Model file for the job. Use its own axes, mm. Round coordinates to 2 decimals unless told otherwise and drop trailing zeros. Loops run counter-clockwise (first coordinate to the right, second up) from the corner with the lowest first, then second, coordinate; pieces in that order, holes last. Notation, with made-up numbers: (-32.5, 30) - (-16.5, 30) arc R20 cw to (-16.5, 64) - close; hole circle Ø2 at (88, 4). An arc over 180 degrees is marked (long way). Answer as a JSON object with one key per item and string values.
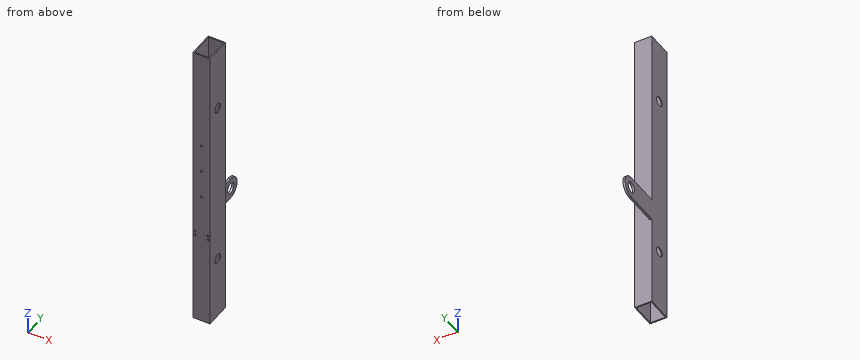
from build123d import *

# Parameters (mm, degrees)
SKETCH1_W           = 50.8
SKETCH1_H           = 76.2
SKETCH1_W_2         = 44.45
SKETCH1_H_2         = 69.85
BOSS_EXTRUDE1_DEPTH = 965.2
CUT_EXTRUDE1_REACH  = 969.287
SKETCH4_R           = 14.224
SKETCH5_R           = 3.175
CUT_EXTRUDE2_DEPTH  = 3.175
CUT_EXTRUDE3_REACH  = 969.287
SKETCH6_W           = 84.151951589
SKETCH6_H           = 76.2
SKETCH7_R           = 15.875
BOSS_EXTRUDE2_DEPTH = 6.35


with BuildPart() as part:
    # Sketch1 → Boss-Extrude1 (new body)
    with BuildSketch(Plane.XY):
        Rectangle(SKETCH1_W, SKETCH1_H)
        Rectangle(SKETCH1_W_2, SKETCH1_H_2, mode=Mode.SUBTRACT)
    extrude(amount=BOSS_EXTRUDE1_DEPTH)

    # Cut-Extrude1: up to this face of the body (flat: up to its plane)
    cut_extrude1_end = Plane(part.part.faces().sort_by_distance((-25.4, 0, 482.6))[0])
    # Sketch4 → Cut-Extrude1 (cut, up to the picked face)
    with BuildSketch(Plane(origin=(25.4, 0, 0), x_dir=(0, 0, -1), z_dir=(1, 0, 0)), mode=Mode.PRIVATE) as cut_extrude1_sk1:
        with Locations(Location((-690.548048411, 0, 0), (0, 0, 90))):
            Circle(SKETCH4_R)
    cut_extrude1_tool1 = split(extrude(cut_extrude1_sk1.sketch, amount=-CUT_EXTRUDE1_REACH, mode=Mode.PRIVATE), bisect_by=cut_extrude1_end, keep=Keep.BOTH, mode=Mode.PRIVATE)
    # Sketch4 → Cut-Extrude1 (cut, up to the picked face)
    with BuildSketch(Plane(origin=(25.4, 0, 0), x_dir=(0, 0, -1), z_dir=(1, 0, 0)), mode=Mode.PRIVATE) as cut_extrude1_sk2:
        with Locations(Location((-190.549048411, 0, 0), (0, 0, 90))):
            Circle(SKETCH4_R)
    cut_extrude1_tool2 = split(extrude(cut_extrude1_sk2.sketch, amount=-CUT_EXTRUDE1_REACH, mode=Mode.PRIVATE), bisect_by=cut_extrude1_end, keep=Keep.BOTH, mode=Mode.PRIVATE)
    add(cut_extrude1_tool1.solids().sort_by(Axis((25.4, 0, 690.548048), (-1, 0, 0)))[0], mode=Mode.SUBTRACT)
    add(cut_extrude1_tool2.solids().sort_by(Axis((25.4, 0, 190.549048), (-1, 0, 0)))[0], mode=Mode.SUBTRACT)

    # Sketch5 → Cut-Extrude2 (cut)
    with BuildSketch(Plane.XZ.offset(38.1)):
        with Locations(Location((-19.05, 276.86, 0), (0, 0, 270))):
            Circle(SKETCH5_R)
        with Locations(Location((-19.05, 289.56, 0), (0, 0, 270))):
            Circle(SKETCH5_R)
        with Locations((19.05, 276.86)):
            Circle(SKETCH5_R)
        with Locations((19.05, 289.56)):
            Circle(SKETCH5_R)
        with Locations(Location((0, 410.718, 0), (0, 0, 270))):
            Circle(SKETCH5_R)
        with Locations(Location((0, 580.898, 0), (0, 0, 270))):
            Circle(SKETCH5_R)
        with Locations(Location((0, 495.808, 0), (0, 0, 270))):
            Circle(SKETCH5_R)
    extrude(amount=-CUT_EXTRUDE2_DEPTH, mode=Mode.SUBTRACT)

    # Cut-Extrude3: up to this face of the body (flat: up to its plane)
    cut_extrude3_end = Plane(part.part.faces().sort_by_distance((-25.4, 0, 483.339612352))[0])
    # Sketch6 → Cut-Extrude3 (cut, up to the picked face)
    with BuildSketch(Plane(origin=(25.4, 0, 0), x_dir=(0, 0, -1), z_dir=(1, 0, 0)), mode=Mode.PRIVATE) as cut_extrude3_sk1:
        with Locations((-923.124024206, 0)):
            Rectangle(SKETCH6_W, SKETCH6_H)
    cut_extrude3_tool1 = split(extrude(cut_extrude3_sk1.sketch, amount=-CUT_EXTRUDE3_REACH, mode=Mode.PRIVATE), bisect_by=cut_extrude3_end, keep=Keep.BOTH, mode=Mode.PRIVATE)
    add(cut_extrude3_tool1.solids().sort_by(Axis((25.4, 0, 923.124024), (-1, 0, 0)))[0], mode=Mode.SUBTRACT)

    # Sketch7 → Boss-Extrude2 (add)
    with BuildSketch(Plane.ZY.offset(25.4)):
        with BuildLine():
            Line((336.55, 139.7), (336.55, 38.1))
            Line((336.55, 38.1), (273.05, 38.1))
            Line((273.05, 38.1), (273.05, 139.7))
            ThreePointArc((273.05, 139.7), (304.8, 171.45), (336.55, 139.7))
        make_face()
        with Locations(Location((304.8, 139.7, 0), (0, 0, 270))):
            Circle(SKETCH7_R, mode=Mode.SUBTRACT)
    extrude(amount=-BOSS_EXTRUDE2_DEPTH)


solid = part.part
1) Drop flat-ended pins along their axis: P1, Ø5, axis at x = 0, z = 495.808, coming from the -Y side (3 decimals); P2, Ø8.5, axis at x = -19.05, z = 289.56, coming from the +Y side; P3, Ø7, axis at x = -21.5, y = 91.5, coming from the +Z side. Give the stop position or say it passes through.
Values follow:
{"P1": "y = 34.925", "P2": "y = 169.49", "P3": "z = 336.55"}
2) Probe probe 1 along Z at (x, y) = (-23.8, 0); probe 2 along Z at (x, y) = (19.05, -37.1) (3 decimals); probe 3 along X at (y, z) = (-35, 276). List the from-to ranges inside material, lowest first.
Values follow:
{"probe 1": "0 to 176.33, 204.77 to 676.32, 704.77 to 881.05", "probe 2": "0 to 273.685, 280.035 to 286.385, 292.735 to 881.048", "probe 3": "-25.4 to -22.11, -15.99 to 15.99, 22.11 to 25.4"}
3) Slice it at A-A on y = 0. List the corners of the cut face in (x, z) (3 decimals), then the cut area to 3 significant figures.
Values follow:
{"outline": "(-25.4, 0) - (-22.225, 0) - (-22.225, 176.325) - (-25.4, 176.325) - close; (-25.4, 204.773) - (-22.225, 204.773) - (-22.225, 676.324) - (-25.4, 676.324) - close; (-25.4, 704.772) - (-22.225, 704.772) - (-22.225, 881.048) - (-25.4, 881.048) - close; (22.225, 0) - (25.4, 0) - (25.4, 176.325) - (22.225, 176.325) - close; (22.225, 204.773) - (25.4, 204.773) - (25.4, 676.324) - (22.225, 676.324) - close; (22.225, 704.772) - (25.4, 704.772) - (25.4, 881.048) - (22.225, 881.048) - close", "area": "5,230 mm²"}
4) Slice it at B-B on z = 358.5. List the corners of the cut face in (x, y) (3 decimals).
Values follow:
{"outline": "(-25.4, -38.1) - (25.4, -38.1) - (25.4, 38.1) - (-25.4, 38.1) - close; hole (-22.225, -34.925) - (22.225, -34.925) - (22.225, 34.925) - (-22.225, 34.925) - close"}
5) Slice it at C-C on y = 73. List the corners of the cut face in (x, z), then the cut area to 3 significant figures.
Values follow:
{"outline": "(-25.4, 273.05) - (-19.05, 273.05) - (-19.05, 336.55) - (-25.4, 336.55) - close", "area": "403 mm²"}
